Autodesk Inventor part; units mm, degrees
ref_plane "YZ Plane" through (0, 0, 0) normal (1, 0, 0) x (0, 1, 0)
ref_plane "XZ Plane" through (0, 0, 0) normal (0, 1, 0) x (-1, 0, 0)
ref_plane "XY Plane" through (0, 0, 0) normal (0, 0, 1) x (1, 0, 0)
sketch "Sketch1" plane through (0, 0, 0) normal (0, 0, 1) x (1, 0, 0)
  line L0 (-85, -15) -> (85, -15)
  line L1 (85, -15) -> (85, 15)
  line L2 (85, 15) -> (-85, 15)
  line L3 (-85, 15) -> (-85, -15)
  line L4 (-85, -15) -> (85, 15) construction
  line L5 (85, -15) -> (-85, 15) construction
  point P0 (0, 0)
  dimension "d0" = 170
  dimension "d1" = 30
extrude "Extrusion1" add sketch "Sketch1" along normal blind 8
sketch "Sketch2" plane through (-85, 15, 0) normal (0, 1, 0) x (1, 0, 0)
  line L0 (170, 0) -> (0, 0) construction
  line L1 (0, 0) -> (0, -8) construction
  line L2 (170, -8) -> (0, -8) construction
  line L3 (170, 0) -> (170, -8) construction
  line L4 (0, -8) -> (0, 0)
  line L5 (85, 0) -> (85, -8) construction
  line L6 (0, 0) -> (4.6188, -8)
  line L7 (0, -8) -> (4.6188, -8)
  line L8 (170, -8) -> (170, 0)
  line L9 (170, 0) -> (165.3812, -8)
  line L10 (170, -8) -> (165.3812, -8)
  point P0 (1.7321, 0)
  dimension "d7" = 30
extrude "Extrusion3" cut sketch "Sketch2" against normal through all
sketch "Sketch3" plane through (-85, -15, 0) normal (-0.866, 0, 0.5) x (0.5, 0, 0.866)
  line L0 (9.2376, 0) -> (0, 0) construction
  line L1 (9.2376, 30) -> (9.2376, 0) construction
  line L2 (0, 30) -> (9.2376, 30) construction
  line L3 (0, 30) -> (0, 0) construction
  line L4 (9.2376, 30) -> (0, 30)
  line L5 (9.2376, 30) -> (9.2376, 20.7624)
  line L6 (0, 0) -> (9.2376, 0)
  line L7 (0, 0) -> (0, 9.2376)
  line L8 (9.2376, 30) -> (9.2376, 0)
  line L9 (9.2376, 20.7624) -> (4.3376, 20.7624)
  line L10 (4.3376, 20.7624) -> (4.3376, 25.1)
  line L11 (4.3376, 25.1) -> (0, 25.1)
  line L12 (0, 30) -> (0, 25.1)
  line L13 (0, 9.2376) -> (4.9, 9.2376)
  line L14 (4.9, 9.2376) -> (4.9, 4.9)
  line L15 (4.9, 4.9) -> (9.2376, 4.9)
  line L16 (9.2376, 0) -> (9.2376, 4.9)
  point P0 (42.5, 15)
  point P1 (4.6188, 30)
  point P2 (9.2376, 15)
  point P3 (4.6188, 30)
  point P4 (9.2376, 15)
  dimension "d15" = 4.9
  dimension "d16" = 4.9
  dimension "d17" = 4.9
  dimension "d18" = 4.9
extrude "Extrusion4" add sketch "Sketch3" along normal blind 3
sketch "Sketch4" plane through (-85, -5.7624, 0) normal (-0.866, 0, 0.5) x (0.5, 0, 0.866)
  line L0 (4.9, -4.3376) -> (9.2376, -4.3376)
  line L1 (9.2376, 11.5248) -> (9.2376, -4.3376)
  line L2 (9.2376, 11.5248) -> (4.3376, 11.5248)
  line L3 (4.3376, 11.5248) -> (4.3376, 15.8624)
  line L4 (4.3376, 15.8624) -> (0, 15.8624)
  line L5 (0, 15.8624) -> (0, 0)
  line L6 (0, 0) -> (4.9, 0)
  line L7 (4.9, 0) -> (4.9, -4.3376)
  point P0 (42.5, 5.7624)
extrude "Extrusion5" cut sketch "Sketch4" against normal blind 3
sketch "Sketch6" plane through (85, -15, 0) normal (0.866, 0, 0.5) x (0.5, 0, -0.866)
  line L0 (0, 0) -> (-9.2376, 0) construction
  line L1 (0, 0) -> (0, 30) construction
  line L2 (-9.2376, 30) -> (0, 30) construction
  line L3 (-9.2376, 0) -> (-9.2376, 30) construction
  line L4 (0, 0) -> (-9.2376, 0)
  line L5 (-9.2376, 0) -> (-9.2376, 9.2376)
  line L6 (-9.2376, 9.2376) -> (-4.3376, 9.2376)
  line L7 (-4.3376, 9.2376) -> (-4.3376, 4.9)
  line L8 (-4.3376, 4.9) -> (0, 4.9)
  line L9 (0, 0) -> (0, 4.9)
  line L10 (0, 0) -> (0, 30)
  line L11 (0, 30) -> (-9.2376, 30)
  line L12 (-9.2376, 25.1) -> (-9.2376, 30)
  line L13 (-9.2376, 25.1) -> (-4.9, 25.1)
  line L14 (-4.9, 25.1) -> (-4.9, 20.7624)
  line L15 (-4.9, 20.7624) -> (0, 20.7624)
  line L16 (0, 20.7624) -> (0, 30)
  point P0 (-42.5, 15)
  point P1 (-7.0688, 25.1)
  dimension "d24" = 4.9
  dimension "d25" = 4.9
  dimension "d26" = 4.9
  dimension "d27" = 4.9
extrude "Extrusion7" add sketch "Sketch6" along normal blind 3
sketch "Sketch7" plane through (85, -10.1, 0) normal (0.866, 0, 0.5) x (0.5, 0, -0.866)
  line L0 (-4.9, 20.2) -> (-9.2376, 20.2)
  line L1 (-9.2376, 4.3376) -> (-9.2376, 20.2)
  line L2 (-9.2376, 4.3376) -> (-4.3376, 4.3376)
  line L3 (-4.3376, 4.3376) -> (-4.3376, 0)
  line L4 (-4.3376, 0) -> (0, 0)
  line L5 (0, 0) -> (0, 15.8624)
  line L6 (0, 15.8624) -> (-4.9, 15.8624)
  line L7 (-4.9, 15.8624) -> (-4.9, 20.2)
  point P0 (-42.5, 10.1)
extrude "Extrusion8" cut sketch "Sketch7" against normal blind 3
sketch "Sketch5" plane through (-85, -15, 0) normal (0, -1, 0) x (1, 0, 0)
  line L0 (4.6188, 8) -> (165.3812, 8) construction
  line L1 (4.6188, 8) -> (2.0207, 9.5) construction
  line L2 (-2.5981, 1.5) -> (2.0207, 9.5) construction
  line L3 (0, 0) -> (-2.5981, 1.5) construction
  line L4 (0, 0) -> (170, 0) construction
  line L5 (0, 0) -> (-2.5981, 1.5)
  line L6 (-1.7321, 3) -> (-2.5981, 1.5)
  line L7 (0, 0) -> (-1.7321, 3)
  line L8 (170, 0) -> (172.5981, 1.5)
  line L9 (167.9793, 9.5) -> (172.5981, 1.5)
  line L10 (165.3812, 8) -> (167.9793, 9.5)
  line L11 (170, 0) -> (171.7321, 3)
  line L12 (171.7321, 3) -> (172.5981, 1.5)
  line L13 (172.5981, 1.5) -> (170, 0)
  point P0 (85, 0)
  dimension "d21" = 30
  dimension "d32" = 30
extrude "Extrusion6" cut sketch "Sketch5" against normal through all
sketch "Sketch9" plane through (0, 0, 8) normal (0, 0, 1) x (1, 0, 0)
  line L0 (80.3812, -15) -> (80.3812, -5.7624) construction
  line L1 (80.3812, -5.7624) -> (80.3812, 10.1) construction
  line L2 (80.3812, 10.1) -> (80.3812, 15) construction
  line L3 (80.3812, 15) -> (-80.3812, 15) construction
  line L4 (-80.3812, 15) -> (-80.3812, 5.7624) construction
  line L5 (-80.3812, 5.7624) -> (-80.3812, -10.1) construction
  line L6 (-80.3812, -10.1) -> (-80.3812, -15) construction
  line L7 (-80.3812, -15) -> (80.3812, -15) construction
  line L8 (49.5, -10) -> (-49.5, -10)
  line L9 (-49.5, -10) -> (-49.5, 10)
  line L10 (-49.5, 10) -> (49.5, 10)
  line L11 (49.5, 10) -> (49.5, -10)
  line L12 (49.5, -10) -> (-49.5, 10) construction
  line L13 (-49.5, -10) -> (49.5, 10) construction
  line L14 (73.5, -10) -> (53.5, -10) construction
  line L15 (53.5, -10) -> (53.5, 10) construction
  line L16 (53.5, 10) -> (73.5, 10) construction
  line L17 (73.5, 10) -> (73.5, -10) construction
  line L18 (63.5, -10) -> (63.5, 10) construction
  line L19 (53.5, 0) -> (73.5, 0) construction
  line L20 (69.5, -6) -> (57.5, -6) construction
  line L21 (57.5, -6) -> (57.5, 6) construction
  line L22 (57.5, 6) -> (69.5, 6) construction
  line L23 (69.5, 6) -> (69.5, -6) construction
  line L24 (69.5, -6) -> (57.5, 6) construction
  line L25 (57.5, -6) -> (69.5, 6) construction
  line L26 (69.5, -6) -> (65.5, -6)
  line L27 (65.5, -6) -> (65.5, 6)
  line L28 (65.5, 6) -> (69.5, 6)
  line L29 (69.5, 6) -> (69.5, -6)
  line L30 (57.5, -6) -> (61.5, -6)
  line L31 (61.5, -6) -> (61.5, 6)
  line L32 (61.5, 6) -> (57.5, 6)
  line L33 (57.5, 6) -> (57.5, -6)
  line L34 (0, -10) -> (0, 10) construction
  line L35 (-69.5, -6) -> (-57.5, -6) construction
  line L36 (-57.5, -6) -> (-57.5, 6) construction
  line L37 (-57.5, 6) -> (-69.5, 6) construction
  line L38 (-69.5, 6) -> (-69.5, -6) construction
  line L39 (-69.5, -6) -> (-57.5, 6) construction
  line L40 (-57.5, -6) -> (-69.5, 6) construction
  line L41 (-69.5, -6) -> (-65.5, -6)
  line L42 (-65.5, -6) -> (-65.5, 6)
  line L43 (-65.5, 6) -> (-69.5, 6)
  line L44 (-69.5, 6) -> (-69.5, -6)
  line L45 (-57.5, -6) -> (-61.5, -6)
  line L46 (-61.5, -6) -> (-61.5, 6)
  line L47 (-61.5, 6) -> (-57.5, 6)
  line L48 (-57.5, 6) -> (-57.5, -6)
  point P0 (0, 0)
  point P1 (49.5, 0)
  point P2 (63.5, 0)
  point P3 (-63.5, 0)
  dimension "d53" = 99
  dimension "d54" = 20
  dimension "d55" = 20
  dimension "d56" = 20
  dimension "d57" = 4
  dimension "d58" = 12
  dimension "d60" = 4
  dimension "d61" = 12
  dimension "d62" = 4
  dimension "d63" = 12
extrude "Extrusion10" cut sketch "Sketch9" against normal through all
properties part number "base"
For this review, take the finished solid that the model builds, in its own axes (mm). A direction names the side the tool comes from. Give positions to 0.01 mm unless a question says otherwise; leave off trailing zeros. Write each loop counter-clockwise with the first axis right and the second up, starting at its lowest first coordinate (ties: lowest second). Pieces come first, ordered by that corner, then holes. Notation, with made-up numbers: M 21.5,73.25 L 58.5,73.25 A22 ccw 58.5,93.25 Z; hole C 15,11.5 d6. An arc over 180 degrees is marked long. One line per item, written item: value.
1) The part is to be moulded in two halves that separate along Y. For faces 4 (the flat face through (-85.3, -11.34, 5.48)), 5 (the flat face through (1, 15, 5)), 6 (the flat face through (61.5, 0, 4)), 7 (the flat face through (-69.5, 0, 4)), say which applies: +Y half, -Y half, draft (parallel to the pull), parting line (faces both ways), or undercut.
Results are:
face 4: draft
face 5: +Y half
face 6: undercut
face 7: undercut
2) For faces 1 (the flat face through (85.854, -12.584, 1.479)), 2 (the flat face through (-68, -6, 4)), 3 (the flat face through (82, -5.762, 6)), list the 3-axis set-ups (+Z, -Z, +X, -X, +Y, -Y) from which the entire face can be reached by the end or side of a thin tool; tool diameter is ignored.
Results are:
face 1: -Z, +X, +Y, -Y
face 2: +Z, -Z
face 3: +X
3) Take a section at C-C, the plane y = 0.5. Write out the cut boundary in (x, z).
Results are:
outline: M -81.53,0 L -69.5,0 L -69.5,8 L -80.38,8 L -77.78,6.5 Z; M -65.5,0 L -61.5,0 L -61.5,8 L -65.5,8 Z; M -57.5,0 L -49.5,0 L -49.5,8 L -57.5,8 Z; M 49.5,0 L 57.5,0 L 57.5,8 L 49.5,8 Z; M 61.5,0 L 65.5,0 L 65.5,8 L 61.5,8 Z; M 69.5,0 L 81.53,0 L 77.78,6.5 L 80.38,8 L 69.5,8 Z
4) For P1, Ø6, axis at x = -14.5, y = -8.5, coming from the -Z side; P2, Ø1, axis at y = -8, z = 5.5, coming from the +X side; P3, Ø4, axis at y = 1, z = 2.5, coming from the +X side; P4, Ø4, axis at y = -0.5, z = 4.5, coming from the +X side, all flat-tipped, find the tip position at first contact; note any pin that passes through.
Results are:
P1: stops at z = 0
P2: stops at x = 85.43
P3: stops at x = 81.24
P4: stops at x = 80.09
5) Take a section at D-D, the plane x = 73. Write out the cut boundary in (y, z), then the cut area to 3 significant figures.
Results are:
outline: M -15,0 L 15,0 L 15,8 L -15,8 Z
area: 240 mm²
6) For line 1 (Y direction, x = 59.5, z = 6.5); line 2 (X direction, y = -7.25, z = 4.75); line 3 (X direction, y = -9, z = 5), list the stretches that pass through material, from the lowest coordinate up. Write a range as from..to.
Results are:
line 1: y = -15..-6, 6..15
line 2: x = -85.72..-83.43, -78.79..-49.5, 49.5..84.55
line 3: x = -85.58..-83.86, -78.65..-49.5, 49.5..84.99
7) Take a section at B-B, the plane x = 43. Write out the cut boundary in (y, z).
Results are:
outline: M -15,0 L -10,0 L -10,8 L -15,8 Z; M 10,0 L 15,0 L 15,8 L 10,8 Z
8) Take a section at A-A, the plane y = -8.5. Write out the cut boundary in (x, z), then the cut area to 3 significant figures.
Results are:
outline: M -86.73,3 L -85,0 L -49.5,0 L -49.5,8 L -80.38,8 L -77.78,6.5 L -79.95,2.74 L -85.15,5.74 Z; M 49.5,0 L 81.53,0 L 80.23,2.26 L 85.43,5.26 L 82.98,9.5 L 80.38,8 L 49.5,8 Z
area: 534 mm²
